Autodesk Inventor part; units mm, degrees
ref_plane "YZ Plane" through (0, 0, 0) normal (1, 0, 0) x (0, 1, 0)
ref_plane "XZ Plane" through (0, 0, 0) normal (0, 1, 0) x (-1, 0, 0)
ref_plane "XY Plane" through (0, 0, 0) normal (0, 0, 1) x (1, 0, 0)
sketch "Sketch1" plane through (0, 0, 0) normal (0, 1, 0) x (-1, 0, 0)
  circle A0 centre (0, 0) radius 3.15
  dimension "d0" = 6.3
extrude "Extrusion1" add sketch "Sketch1" along normal blind 12
sketch "Sketch2" plane through (0, 12, 0) normal (0, 1, 0) x (1, 0, 0)
  circle A0 centre (0, 0) radius 3.15
  circle A1 centre (0, 0) radius 3.9
  dimension "d3" = 7.8
extrude "Extrusion2" add sketch "Sketch2" along normal blind 6 contours A0 | A1
chamfer "Chamfer1" distance 0.75 angle 45 1 edges at (-3.9, 12, 0)
sketch "Sketch3" plane through (0, 18, 0) normal (0, 1, 0) x (1, 0, 0)
  circle A0 centre (0, 0) radius 3.9
  circle A1 centre (0, 0) radius 5
  dimension "d9" = 10
extrude "Extrusion3" add sketch "Sketch3" along normal blind 286 contours A0 | A1
sketch "Sketch4" plane through (0, 304, 0) normal (0, 1, 0) x (1, 0, 0)
  circle A0 centre (0, 0) radius 5
  circle A1 centre (0, 0) radius 3.9
  dimension "d12" = 7.8
extrude "Extrusion4" add sketch "Sketch4" along normal blind 10 contours A1
chamfer "Chamfer2" distance 0.5 angle 45 2 edges at (-3.9, 314, 0) (3.15, 0, 0)
thread "Thread1"
properties part number "ZACMEScrew" material "Steel"
Design review of the part built by this model. Coordinates are the model's own, in mm. A direction names the side the tool comes from. Give positions to 0.01 mm unless a question says otherwise; leave off trailing zeros. Order: outer loops, then holes, each group sorted by start corner. A loop starts at its lowest first (then second) coordinate and runs counter-clockwise, first axis right, second up. Notation, with made-up numbers: (8, 17.25) - (61, 17.25) arc R33 ccw to (61, 49.25) - close; hole circle Ø7 at (47, 1). An arc over 180 degrees is marked (long way). Write item = value, one per line. Start each with the question number.
Q1. Tool access review of faces 1 (the face through (-2.87, 308.68, 2.64)), 2 (the face through (3, 18, 3)), 3 (the face through (0, 0, 0)): name each direction out of +Z, -Z, +X, -X, +Y, -Y from which nothing blocks a thin tool from reaching the whole face with its end or side.
Q2. Clearance check with flat-ended pins moving along their axes: pin 1 Ø5 at (x, y) = (3.5, 152.5) entering from +Z; pin 2 Ø3 at (x, y) = (-3.5, 160) entering from -Z; pin 3 Ø5 at (y, z) = (138.5, 3.5) entering from -X. State where each tip first meets the part, or that it passes through.
Q3. We need section C-C on y = 243. State the section outline as (x, z) points.
Q4. To check wall thickness, follow L1, parallel to Y at x = -2, z = -4.5; L2, parallel to Z at x = -4.25, y = 56; L3, parallel to X at y = 258, z = 4. State the ranges of each line that lie inside material, in increasing order. Write a range as from..to.
Working result:
q1.face_1 = +Y
q1.face_2 = -Y
q1.face_3 = +Z, -Z, +X, -X, -Y
q2.pin_1 = 4.9
q2.pin_2 = -4.58
q2.pin_3 = -4.9
q3.outline = circle Ø10 at (0, 0)
q4.L1 = 18..304
q4.L2 = -2.63..2.63
q4.L3 = -3..3
